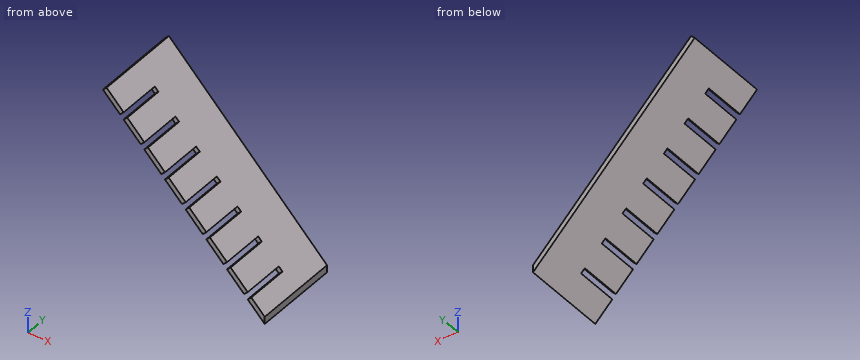
from build123d import *

# Parameters (mm, degrees)
F1_DEPTH = 152.4
F2_W     = 19.05
F2_H     = 152.4
F3_DEPTH = 19.05


with BuildPart() as f1:
    # F0 (on Front) → F1 (new body, symmetric)
    with BuildSketch(Plane.XZ):
        Polygon((-218.657332487, 731.8369923304), (378.5296995641, 134.6499602793), (378.5296995641, 161.5907286425), (-205.1869483054, 745.307376512), align=None)
    extrude(amount=F1_DEPTH, both=True)

    # F2 (on face) → F3 (cut)
    with BuildSketch(Plane(origin=(270.0602141033, 0, 270.0602141033), x_dir=(0.7071067812, 0, -0.7071067812), z_dir=(0.7071067812, 0, 0.7071067812))):
        with Locations((74.0240174423, -76.2)):
            Rectangle(F2_W, F2_H)
        with Locations((-33.9259825577, -76.2)):
            Rectangle(F2_W, F2_H)
        with Locations((-141.8759825577, -76.2)):
            Rectangle(F2_W, F2_H)
        with Locations((-249.8259825577, -76.2)):
            Rectangle(F2_W, F2_H)
        with Locations((-357.7759825577, -76.2)):
            Rectangle(F2_W, F2_H)
        with Locations((-465.7259825577, -76.2)):
            Rectangle(F2_W, F2_H)
        with Locations((-573.6759825577, -76.2)):
            Rectangle(F2_W, F2_H)
    extrude(amount=-F3_DEPTH, mode=Mode.SUBTRACT)


solid = f1.part
Read the model definition and answer for the solid it produces. Units are mm, in the model's axes. Coordinates: 2 decimals unless noted, no trailing zeros. Loops run counter-clockwise (first coordinate to the right, second up) from the corner with the lowest first, then second, coordinate; pieces in that order, holes last. Notation, with made-up numbers: (23, -1) - (70, -1) arc R27 ccw to (70, 19) - close; hole circle Ø7 at (-38.5, 40). An arc over 180 degrees is marked (long way). Answer in a Markdown table with one row per item.
Q1. Given P1, Ø4, axis at y = 84.5, z = 659, coming from the +X side; P2, Ø13.5, axis at x = 240.5, z = 291.5, coming from the -Y side; P3, Ø3, axis at y = 115.5, z = 597.5, coming from the +X side, each flat-ended and moving along its own axis, determine where each tip first touches the part or whether it passes through.
Here are the results:
| item | result |
|---|---|
| P1 | stops at x = -116.88 |
| P2 | stops at y = 0 |
| P3 | stops at x = -55.88 |
Q2. Straight lines are drawn through the part: line 1 along Y through (x, z) = (164, 352.5); line 2 along Z through (x, y) = (256, 81); line 3 along Z through (x, y) = (252.5, 123). For each, find the intervals that lie inside material, in ascending order. Write a range as [from, to].
Here are the results:
| item | result |
|---|---|
| line 1 | y = [0, 152.4] |
| line 2 | z = [257.18, 284.12] |
| line 3 | z = [260.68, 287.62] |
Q3. Find section C-C on x = 196.5. Write down the section's boundary in (y, z), plus the area to 3 significant figures.
Here are the results:
| item | result |
|---|---|
| outline | (-152.4, 316.68) - (152.4, 316.68) - (152.4, 343.62) - (-152.4, 343.62) - close |
| area | 8,210 mm^2 |
Q4. Find section B-B on y = 73. Write down the section's boundary in (x, z), plus the area to 3 significant figures.
Here are the results:
| item | result |
|---|---|
| outline | (-218.66, 731.84) - (378.53, 134.65) - (378.53, 161.59) - (-205.19, 745.31) - close |
| area | 15,900 mm^2 |
Q5. Find section A-A on y = -27. Count the separate pieces of the cut face and the enclosed holes in it, plus the area to 3 significant figures.
Here are the results:
| item | result |
|---|---|
| separate pieces | 8 |
| enclosed holes | 0 |
| area | 13,400 mm^2 |
